Can you work these out from the model? Positions are in its coordinate system, mm. A direction names the side the tool comes from. Give positions to 0.01 mm unless a question says otherwise; leave off trailing zeros. Loops run counter-clockwise (first coordinate to the right, second up) from the corner with the lowest first, then second, coordinate; pieces in that order, holes last. Notation, with made-up numbers: M -26.75,-19.5 L 21.25,-19.5 A23 ccw 21.25,13.5 Z; hole C 29,-34 d7. An arc over 180 degrees is marked long. Use CSV: the item, a comma, the result in double quotes.
from build123d import *

# Parameters (mm, degrees)
F0_W      = 120
F0_H      = 38
F1_DEPTH  = 2
F2_W      = 70
F2_H      = 2.5
F3_DEPTH  = 5
F5_D      = 2.3
F5_DEPTH  = 5
F6_R      = 3.5
F3_FACE_R = 1.15
F7_ANGLE  = -7.5


with BuildPart() as f1:
    # F0 (on Top) → F1 (new body)
    with BuildSketch(Plane.XY):
        Rectangle(F0_W, F0_H)
    extrude(amount=F1_DEPTH)

    # F2 (on face) → F3 (join)
    with BuildSketch(Plane.XY.offset(2)):
        with Locations((0, -17.75)):
            Rectangle(F2_W, F2_H)
    extrude(amount=F3_DEPTH)

    # F5
    with Locations(Plane.XZ.offset(19)):
        with Locations((-30, 4.5), (-15, 4.5), (0, 4.5), (15, 4.5), (30, 4.5)):
            Hole(F5_D / 2, depth=F5_DEPTH)

    # F6
    f6_edges = [f1.edges().sort_by_distance(p)[0] for p in [
        (-60, -19, 1),
        (-60, 19, 1),
        (60, 19, 1),
        (60, -19, 1),
    ]]
    fillet(f6_edges, radius=F6_R)

    # F3_face (on face) → F7 (revolve)
    with BuildSketch(Plane(origin=(0, -19, 3.076271), x_dir=(1, 0, 0), z_dir=(0, -1, 0))):
        Polygon((-56.5, -3.076271), (56.5, -3.076271), (56.5, -1.076271), (35, -1.076271), (35, 3.923729), (-35, 3.923729), (-35, -1.076271), (-56.5, -1.076271), align=None)
        with Locations((-30, 1.423729)):
            Circle(F3_FACE_R, mode=Mode.SUBTRACT)
        with Locations((-15, 1.423729)):
            Circle(F3_FACE_R, mode=Mode.SUBTRACT)
        with Locations((0, 1.423729)):
            Circle(F3_FACE_R, mode=Mode.SUBTRACT)
        with Locations((15, 1.423729)):
            Circle(F3_FACE_R, mode=Mode.SUBTRACT)
        with Locations((30, 1.423729)):
            Circle(F3_FACE_R, mode=Mode.SUBTRACT)
    revolve(axis=Axis((0, -19, 0), (-1, 0, 0)), revolution_arc=F7_ANGLE)


solid = f1.part
Q1. For faces 1 (the flat face through (-35, -18, 4)), 2 (the flat face through (35, -18, 5)), 3 (the flat face through (-1, 19, 1)), which set-ups out of +Z, -Z, +X, -X, +Y, -Y let a thin tool reach every point of the face, with its end or its side?
Model answer:
face 1,"+Z, -X, +Y, -Y"
face 2,"+Z, +X, +Y, -Y"
face 3,"+Z, -Z, +X, -X, +Y"
Q2. Please list where these lines run through material, in increasing order: L1, parallel to X at y = -17.25, z = 4.5; L2, parallel to Z at x = -30, y = -17.3; L3, parallel to Z at x = -53, y = -4.5. Write a range as from..to.
Model answer:
L1,"-35..-31.15, -28.85..-16.15, -13.85..-1.15, 1.15..13.85, 16.15..28.85, 31.15..35"
L2,"0..3.35, 5.65..7"
L3,"0..2"
Q3. I want a section at B-B, the plane y = -0.5. Please give me the cut outline in (x, z), then the cut area to 3 significant figures.
Model answer:
outline,"M -60,0 L 60,0 L 60,2 L -60,2 Z"
area,"240 mm2"
Q4. If we mould it in two halves opening along X, with no side actions, what happens to faces 4 (the cylindrical face through (15.848, -17.732, 5.277)), 5 (the flat face through (-60, 0, 1)), 6 (the flat face through (0, -16.5, 6))? For each: released by +X, released by -X, zero draft, split by the parting line, or undercut.
Model answer:
face 4,"undercut"
face 5,"released by -X"
face 6,"zero draft"
Q5. I want a section at C-C, the plane x = -52. Please give me the cut outline in (y, z), then the cut area to 3 significant figures.
Model answer:
outline,"M -19.26,1.98 L -19,0 L 19,0 L 19,2 L -19,2 A2 ccw Z"
area,"76.3 mm2"
Q6. I want a section at A-A, the plane x = -30. Please give me the cut outline in (y, z), then the cut area to 3 significant figures.
Model answer:
outline,"M -19.91,6.94 L -19.74,5.6 A5.65 cw -19,5.65 L -16.5,5.65 L -16.5,7 L -19,7 A7 ccw Z; M -19.44,3.32 L -19,0 L 19,0 L 19,2 L -16.5,2 L -16.5,3.35 L -19,3.35 A3.35 ccw Z"
area,"84.6 mm2"
Q7. I want a section at D-D, the plane x = 17.5. Please give me the cut outline in (y, z).
Model answer:
outline,"M -19.91,6.94 L -19,0 L 19,0 L 19,2 L -16.5,2 L -16.5,7 L -19,7 A7 ccw Z"
Q8. I'm going to push flat-ended pins straight in: P1, Ø19, axis at x = -4.5, y = -1.5, coming from the +Z side; P2, Ø1, axis at x = -3, y = -11.5, coming from the -Z side; P3, Ø4, axis at x = 6, z = 5.5, coming from the +Y side; P4, Ø4, axis at y = -17.5, z = 4.5, coming from the +X side. Where does each tip first touch, or does it pass through?
Model answer:
P1,"z = 2"
P2,"z = 0"
P3,"y = -16.5"
P4,"x = 35"
